Design review of the part built by this model. Coordinates are the model's own, in mm. A direction names the side the tool comes from. Give positions to 0.01 mm unless a question says otherwise; leave off trailing zeros. Write each loop counter-clockwise with the first axis right and the second up, starting at its lowest first coordinate (ties: lowest second). Pieces come first, ordered by that corner, then holes. Notation, with made-up numbers: (35, 44.25) -> (94, 44.25) arc R26 cw to (94, 79.25) -> close; hole circle Ø11 at (-26.75, 31). An arc over 180 degrees is marked (long way). Answer as a JSON object with one key per item and string values.
```python
from build123d import *

# Parameters (mm, degrees)
SKETCH1_R           = 1.6
BOSS_EXTRUDE1_DEPTH = 3
SKETCH2_R           = 3.5
SKETCH2_R_2         = 1.6
BOSS_EXTRUDE2_DEPTH = 4.5


with BuildPart() as part:
    # Sketch1 → Boss-Extrude1 (new body)
    with BuildSketch(Plane(origin=(0, 0, 0), x_dir=(1, 0, 0), z_dir=(0, 1, 0))):
        with BuildLine():
            Line((30, -3.5), (-30, -3.5))
            ThreePointArc((-30, -3.5), (-33.5, 0), (-30, 3.5))
            Line((-30, 3.5), (30, 3.5))
            ThreePointArc((30, 3.5), (33.5, 0), (30, -3.5))
        make_face()
        with Locations(Location((-30, 0, 0), (0, 0, 270))):
            Circle(SKETCH1_R, mode=Mode.SUBTRACT)
        with Locations(Location((-10, 0, 0), (0, 0, 270))):
            Circle(SKETCH1_R, mode=Mode.SUBTRACT)
        with Locations(Location((10, 0, 0), (0, 0, 270))):
            Circle(SKETCH1_R, mode=Mode.SUBTRACT)
        with Locations(Location((30, 0, 0), (0, 0, 270))):
            Circle(SKETCH1_R, mode=Mode.SUBTRACT)
    extrude(amount=BOSS_EXTRUDE1_DEPTH)

    # Sketch2 → Boss-Extrude2 (add)
    # profile 1 of 4: a face of its own
    with BuildSketch(Plane(origin=(0, 3, 0), x_dir=(1, 0, 0), z_dir=(0, 1, 0))):
        with Locations(Location((-30, 0, 0), (0, 0, 270))):
            Circle(SKETCH2_R)
        with Locations(Location((-30, 0, 0), (0, 0, 270))):
            Circle(SKETCH2_R_2, mode=Mode.SUBTRACT)
    # profile 2 of 4: a face of its own
    with BuildSketch(Plane(origin=(0, 3, 0), x_dir=(1, 0, 0), z_dir=(0, 1, 0))):
        with Locations(Location((-10, 0, 0), (0, 0, 270))):
            Circle(SKETCH2_R)
        with Locations(Location((-10, 0, 0), (0, 0, 270))):
            Circle(SKETCH2_R_2, mode=Mode.SUBTRACT)
    # profile 3 of 4: a face of its own
    with BuildSketch(Plane(origin=(0, 3, 0), x_dir=(1, 0, 0), z_dir=(0, 1, 0))):
        with Locations(Location((10, 0, 0), (0, 0, 270))):
            Circle(SKETCH2_R)
        with Locations(Location((10, 0, 0), (0, 0, 270))):
            Circle(SKETCH2_R_2, mode=Mode.SUBTRACT)
    # profile 4 of 4: a face of its own
    with BuildSketch(Plane(origin=(0, 3, 0), x_dir=(1, 0, 0), z_dir=(0, 1, 0))):
        with Locations(Location((30, 0, 0), (0, 0, 270))):
            Circle(SKETCH2_R)
        with Locations(Location((30, 0, 0), (0, 0, 270))):
            Circle(SKETCH2_R_2, mode=Mode.SUBTRACT)
    extrude(amount=BOSS_EXTRUDE2_DEPTH)


solid = part.part
```
(1) We need section D-D, the plane x = -20. State the section outline as (y, z) points.
Here are the results:
{"outline": "(0, -3.5) -> (3, -3.5) -> (3, 3.5) -> (0, 3.5) -> close"}
(2) We need section A-A, the plane y = 3.75. State the section outline as (x, z) points.
Here are the results:
{"outline": "circle Ø7 at (-30, 0); circle Ø7 at (-10, 0); circle Ø7 at (10, 0); circle Ø7 at (30, 0); hole circle Ø3.2 at (-30, 0); hole circle Ø3.2 at (-10, 0); hole circle Ø3.2 at (10, 0); hole circle Ø3.2 at (30, 0)"}
(3) Clearance check with flat-ended pins moving along their axes: pin 1 (1 mm diameter, centred on y = 4.5, z = 2, fed in from +X); pin 2 (1 mm diameter, centred on y = 5.5, z = -2, fed in from -X); pin 3 (3.5 mm diameter, centred on x = -15, z = -1, fed in from +Y); pin 4 (2 mm diameter, centred on x = 2, z = -1.5, fed in from +Y). State where each tip first meets the part, or that it passes through.
Here are the results:
{"pin 1": "stops at x = 33.16", "pin 2": "stops at x = -33.16", "pin 3": "stops at y = 7.5", "pin 4": "stops at y = 3"}
(4) For line 1 along X through (y, z) = (1.75, 0); line 2 along X through (y, z) = (3.25, -1.75); line 3 along Y through (x, z) = (14, 2), list the stretches that pass through material, from the lowest coordinate up.
Here are the results:
{"line 1": "x = -33.5 to -31.6, -28.4 to -11.6, -8.4 to 8.4, 11.6 to 28.4, 31.6 to 33.5", "line 2": "x = -33.03 to -26.97, -13.03 to -6.97, 6.97 to 13.03, 26.97 to 33.03", "line 3": "y = 0 to 3"}
(5) We need section B-B, the plane z = 0. Give the number of separate pieces and of enclosed holes in the cut face, then the cut area to 3 significant figures.
Here are the results:
{"separate pieces": "5", "enclosed holes": "0", "area": "231 mm²"}
(6) For faces 1 (the cylindrical face through (8.44, 3.7, -0.35)), 2 (the cylindrical face through (-33.105, 4.531, 1.615)), list the 3-axis set-ups (+Z, -Z, +X, -X, +Y, -Y) from which the entire face can be reached by the end or side of a thin tool; tool diameter is ignored.
Here are the results:
{"face 1": "+Y, -Y", "face 2": "+Y"}
(7) We need section C-C, the plane x = 7.5. State the section outline as (y, z) points.
Here are the results:
{"outline": "(0, -3.5) -> (3, -3.5) -> (3, -2.45) -> (7.5, -2.45) -> (7.5, 2.45) -> (3, 2.45) -> (3, 3.5) -> (0, 3.5) -> close"}
(8) The part is to be moulded in two halves that separate along Z. For faces 3 (the cylindrical face through (31.586, 3.698, -0.208)), 4 (the cylindrical face through (-13.417, 5.219, -0.759)), 5 (the flat face through (20, 3, 0)), 6 (the flat face through (0, 1, -3.5)), say which applies: +Z half, -Z half, draft (parallel to the pull), parting line (faces both ways), or undercut.
Here are the results:
{"face 3": "undercut", "face 4": "parting line", "face 5": "draft", "face 6": "-Z half"}
